```python
from build123d import *

# Parameters (mm, degrees)
SKETCH_1_R                = 40
EXTRUDE_1_DEPTH           = 20
SKETCH_2_R                = 10
EXTRUDE_2_DEPTH           = 60
EXTRUDE_3_DEPTH           = 15
EXTRUDE_3_DEPTH_BACK      = 15
SKETCH_3_R                = 36.590327892
SKETCH_2_2_R              = 10
EXTRUDE_4_DEPTH           = 450
EXTRUDE_5_DEPTH           = 0.0001
EXTRUDE_5_DEPTH_BACK      = 30
SKETCH_7_R                = 30
SKETCH_8_R                = 10
EXTRUDE_6_DEPTH           = 10
EXTRUDE_6_TAPER           = 30
EXTRUDE_6_OTHER_WAY_DEPTH = 0.0001


with BuildPart() as part:
    # Sketch 1 → Extrude 1 (new body)
    with BuildSketch(Plane(origin=(0, 0, 0), x_dir=(1, 0, 0), z_dir=(0, 1, 0))):
        with Locations(Location((0, 0, 0), (0, 0, 270))):
            Circle(SKETCH_1_R)
    extrude(amount=EXTRUDE_1_DEPTH)

    # Sketch 2 → Extrude 2 (add)
    with BuildSketch(Plane(origin=(0, 0, 0), x_dir=(-1, 0, 0), z_dir=(0, -1, 0))):
        with Locations(Location((0, 0, 0), (0, 0, 90))):
            Circle(SKETCH_2_R)
    extrude(amount=EXTRUDE_2_DEPTH)

    # Sketch 3 → Extrude 3 (add, two sides: drawn at the far end of the back side and taken through both)
    with BuildSketch(Plane.XY.offset(-EXTRUDE_3_DEPTH_BACK)):
        with Locations((0, -91.676757002)):
            Circle(SKETCH_3_R)
    extrude(amount=EXTRUDE_3_DEPTH + EXTRUDE_3_DEPTH_BACK)

    # Sketch 2_2 → Extrude 4 (add)
    with BuildSketch(Plane(origin=(0, 0, 0), x_dir=(-1, 0, 0), z_dir=(0, -1, 0))):
        with Locations(Location((0, 0, 0), (0, 0, 270))):
            Circle(SKETCH_2_2_R)
    extrude(amount=EXTRUDE_4_DEPTH)

    # Sketch 7 → Extrude 5 (add, two sides: drawn at the far end of the back side and taken through both)
    with BuildSketch(Plane(origin=(0, 0, -15), x_dir=(-1, 0, 0), z_dir=(0, 0, -1)).offset(-EXTRUDE_5_DEPTH_BACK)):
        with Locations((0, -262.19236229)):
            Circle(SKETCH_7_R)
    extrude(amount=EXTRUDE_5_DEPTH + EXTRUDE_5_DEPTH_BACK)

    # Sketch 8 → Extrude 6 (add)
    with BuildSketch(Plane.XZ.offset(450)):
        with Locations(Location((0, 0, 0), (0, 0, 90))):
            Circle(SKETCH_8_R)
    extrude(amount=EXTRUDE_6_DEPTH, taper=EXTRUDE_6_TAPER)

    # Sketch 8 → Extrude 6 other way (add)
    with BuildSketch(Plane.XZ.offset(450)):
        with Locations(Location((0, 0, 0), (0, 0, 90))):
            Circle(SKETCH_8_R)
    extrude(amount=-EXTRUDE_6_OTHER_WAY_DEPTH)


solid = part.part
```
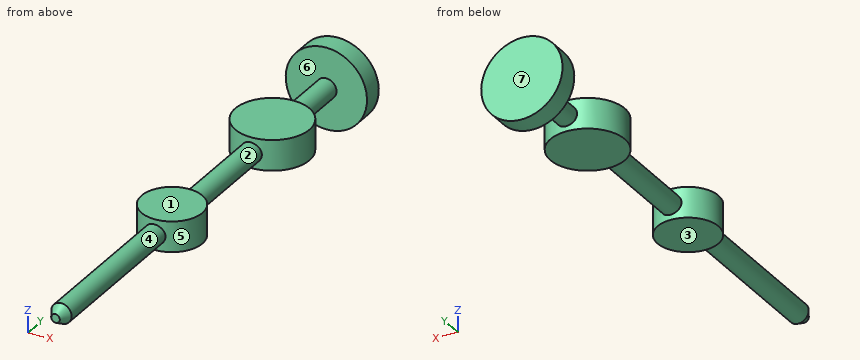
Source: CAD feature listing. Evaluate the final solid. Frame: model axes, mm. Face numbers are marked on the shaded views. A direction names the side the tool comes from. Round coordinates to 2 decimals unless told otherwise and drop trailing zeros. Write each loop counter-clockwise with the first axis right and the second up, starting at its lowest first coordinate (ties: lowest second). Pieces come first, ordered by that corner, then holes. Notation, with made-up numbers: M 33,55 L 44,55 A21 ccw 44,59 Z; hole C 49.5,-31 d6. An arc over 180 degrees is marked long. Use CSV: the item, a comma, the result in double quotes. Start each with the question number.
Q1. Cut plane B-B on x = -26. Output: boundary loops of the cut face in (y, z).
Q2. Access query for the marked faces 1, 2 and 3. Directions: +Z, -Z, +X, -X, +Y, -Y. A direction counts if a zero-diameter tool reaches every point of the face in a straight line with its end or side. Return the directions, or none.
Q3. Line query: line 1 (Y direction, x = 7.5, z = -27); line 2 (Z direction, x = -0.5, y = -268); line 3 (Z direction, x = 6, y = -297.5). Output: solid intervals per line, ascending. Write a range as from..to.
Q4. First-contact query: P1, Ø12, axis at y = -78.5, z = 0, coming from the +X side; P2, Ø12, axis at x = -7.5, y = -94.5, coming from the +Z side; P3, Ø6, axis at y = -219.5, z = 15.5, coming from the +X side (3 decimals); P4, Ø22, axis at x = 10.5, y = -108, coming from the -Z side. Flat tips, straight axial feed; report the tip coordinate or a pass-through.
Q5. Cut plane A-A on z = 0. Output: boundary loops of the cut face in (x, y).
Q6. Cut plane C-C on y = -188.5. Output: boundary loops of the cut face in (x, z), plus the area to 3 significant figures.
Q7. Pull-direction query (Y, two-part tool) for the marked faces 4, 5, 6 and 7; classes: +Y half, -Y half, draft (parallel to the pull), parting line (faces both ways), or undercut.
Q8. Cut plane D-D on x = 23. Output: boundary loops of the cut face in (y, z), plus the area to 3 significant figures.
Results found:
1,outline,"M -277.16,-15 L -247.23,-15 L -247.23,15 L -277.16,15 Z; M -117.42,-15 L -65.93,-15 L -65.93,15 L -117.42,15 Z; M 0,-30.4 L 20,-30.4 L 20,30.4 L 0,30.4 Z"
2,face 1,"+Z, +X, -X, -Y"
2,face 2,"none"
2,face 3,"-Z, +X, -X, -Y"
3,line 1,"0..20"
3,line 2,"-15..15"
3,line 3,"-8..8"
4,P1,"x = 35.88"
4,P2,"z = 15"
4,P3,"through"
4,P4,"z = -15"
5,outline,"M -40,0 L -10,0 L -10,-56.48 A36.59 ccw -10,-126.87 L -10,-233.91 A30 ccw -10,-290.48 L -10,-450 L -4.23,-460 L 4.23,-460 L 10,-450 L 10,-290.48 A30 ccw 10,-233.91 L 10,-126.87 A36.59 ccw 10,-56.48 L 10,0 L 40,0 L 40,20 L -40,20 Z"
6,outline,"C 0,0 d20"
6,area,"314 mm^2"
7,face 4,"draft"
7,face 5,"undercut"
7,face 6,"undercut"
7,face 7,"+Y half"
8,outline,"M -281.45,-15 L -242.93,-15 L -242.93,15 L -281.45,15 Z; M -120.13,-15 L -63.22,-15 L -63.22,15 L -120.13,15 Z; M 0,-32.73 L 20,-32.73 L 20,32.73 L 0,32.73 Z"
8,area,"4,170 mm^2"
